Check sheet for the drawn part. Datum: minimum x, y, z corner. Units: mm. Coordinates: 2 decimals unless noted, no trailing zeros. Write each loop counter-clockwise with the first axis right and the second up, starting at its lowest first coordinate (ties: lowest second). Pieces come first, ordered by that corner, then holes. Notation, with made-up numbers: (79, 40.5) - (114, 40.5) arc R25 ccw to (114, 72.5) - close; hole circle Ø7 at (7, 8). An arc over 180 degrees is marked (long way). Write each question's results on one line, items separated by ' | '.
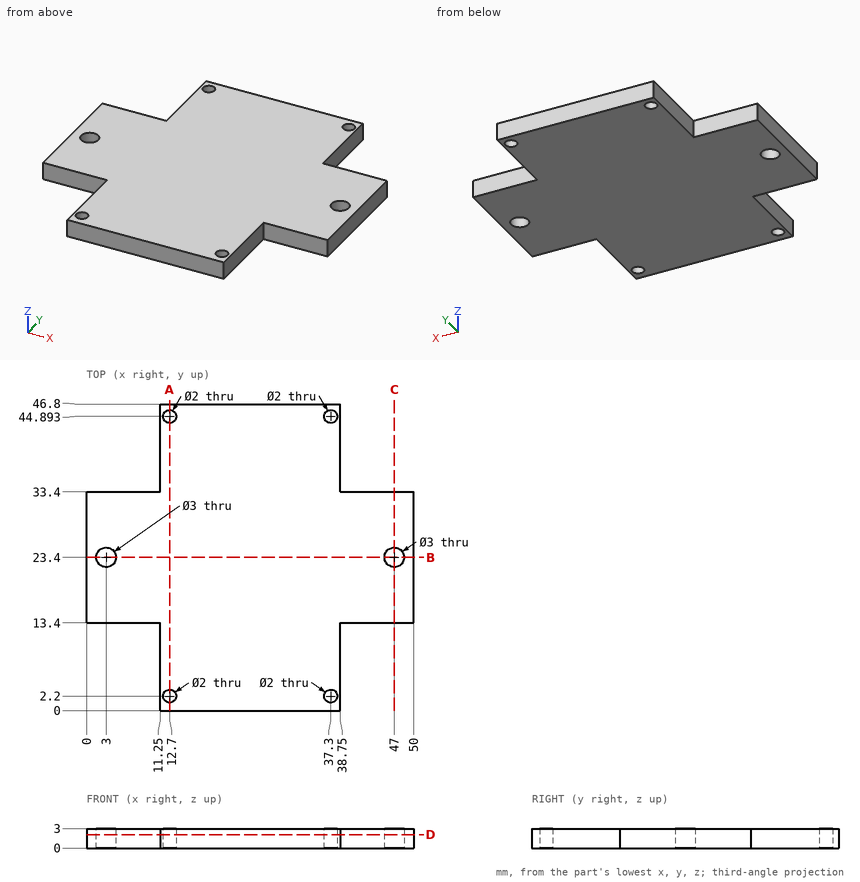
1. Sectioned sample at A-A (x = 12.7). Record the cut outline in (y, z).
Values follow:
outline: (0, 0) - (1.2, 0) - (1.2, 3) - (0, 3) - close; (3.2, 0) - (43.89, 0) - (43.89, 3) - (3.2, 3) - close; (45.89, 0) - (46.8, 0) - (46.8, 3) - (45.89, 3) - close
2. Material ranges on L1, parallel to Y at x = 12.7, z = 1.45; L2, parallel to Y at x = 47, z = 1.75; L3, parallel to X at y = 6.5, z = 1.75, recorded low to high. Write a range as [from, to].
Values follow:
L1: y = [0, 1.2], [3.2, 43.89], [45.89, 46.8] | L2: y = [13.4, 21.9], [24.9, 33.4] | L3: x = [11.25, 38.75]
3. Sectioned sample at D-D (z = 2.05). Record the cut outline in (x, y).
Values follow:
outline: (0, 13.4) - (11.25, 13.4) - (11.25, 0) - (38.75, 0) - (38.75, 13.4) - (50, 13.4) - (50, 33.4) - (38.75, 33.4) - (38.75, 46.8) - (11.25, 46.8) - (11.25, 33.4) - (0, 33.4) - close; hole circle Ø3 at (3, 23.4); hole circle Ø2 at (12.7, 2.2); hole circle Ø2 at (12.7, 44.89); hole circle Ø2 at (37.3, 2.2); hole circle Ø2 at (37.3, 44.89); hole circle Ø3 at (47, 23.4)
4. Sectioned sample at C-C (x = 47). Record the cut outline in (y, z), then the cut area to 3 significant figures.
Values follow:
outline: (13.4, 0) - (21.9, 0) - (21.9, 3) - (13.4, 3) - close; (24.9, 0) - (33.4, 0) - (33.4, 3) - (24.9, 3) - close | area: 51.0 mm^2
5. Sectioned sample at B-B (y = 23.4). Record the cut outline in (x, z), then the cut area to 3 significant figures.
Values follow:
outline: (0, 0) - (1.5, 0) - (1.5, 3) - (0, 3) - close; (4.5, 0) - (45.5, 0) - (45.5, 3) - (4.5, 3) - close; (48.5, 0) - (50, 0) - (50, 3) - (48.5, 3) - close | area: 132 mm^2
6. Go/stop test with flat-tipped pins: pin 1 (0.9 mm diameter, centred on x = 43, z = 2, fed in from -Y); pin 2 (0.9 mm diameter, centred on y = 8, z = 1, fed in from -X); pin 3 (1.5 mm diameter, centred on y = 42, z = 1.5, fed in from +X). Record where each tip stops, or that it passes through.
Values follow:
pin 1: stops at y = 13.4 | pin 2: stops at x = 11.25 | pin 3: stops at x = 38.75
